```python
from build123d import *

# Parameters (mm, degrees)
SKETCH1_W           = 115
SKETCH1_H           = 150
SKETCH1_R           = 7.5
SKETCH1_W_2         = 15
SKETCH1_H_2         = 3
BOSS_EXTRUDE1_DEPTH = 3


with BuildPart() as part:
    # Sketch1 → Boss-Extrude1 (new body)
    with BuildSketch(Plane.XY):
        Rectangle(SKETCH1_W, SKETCH1_H)
        with Locations((0, -13.5)):
            Circle(SKETCH1_R, mode=Mode.SUBTRACT)
        with Locations((15, 70.5)):
            Rectangle(SKETCH1_W_2, SKETCH1_H_2, mode=Mode.SUBTRACT)
        with Locations((-40, 70.5)):
            Rectangle(SKETCH1_W_2, SKETCH1_H_2, mode=Mode.SUBTRACT)
        with Locations((-15, 70.5)):
            Rectangle(SKETCH1_W_2, SKETCH1_H_2, mode=Mode.SUBTRACT)
        with Locations((40, 70.5)):
            Rectangle(SKETCH1_W_2, SKETCH1_H_2, mode=Mode.SUBTRACT)
        with Locations((40, -70.5)):
            Rectangle(SKETCH1_W_2, SKETCH1_H_2, mode=Mode.SUBTRACT)
        with Locations((15, -70.5)):
            Rectangle(SKETCH1_W_2, SKETCH1_H_2, mode=Mode.SUBTRACT)
        with Locations((-15, -70.5)):
            Rectangle(SKETCH1_W_2, SKETCH1_H_2, mode=Mode.SUBTRACT)
        with Locations((-40, -70.5)):
            Rectangle(SKETCH1_W_2, SKETCH1_H_2, mode=Mode.SUBTRACT)
        with Locations((14.7, 43.5)):
            Rectangle(SKETCH1_W_2, SKETCH1_H_2, mode=Mode.SUBTRACT)
        with Locations((-39.7, 43.5)):
            Rectangle(SKETCH1_W_2, SKETCH1_H_2, mode=Mode.SUBTRACT)
        with Locations((-14.7, 43.5)):
            Rectangle(SKETCH1_W_2, SKETCH1_H_2, mode=Mode.SUBTRACT)
        with Locations((39.7, 43.5)):
            Rectangle(SKETCH1_W_2, SKETCH1_H_2, mode=Mode.SUBTRACT)
        with BuildLine():
            Line((39.5, -7.5), (39.5, 11.686291501))
            ThreePointArc((39.5, 11.686291501), (37.648050297, 14.457930099), (34.378679656, 13.807611845))
            Line((34.378679656, 13.807611845), (16.655175669, -3.915892143))
            ThreePointArc((16.655175669, -3.915892143), (16.374485428, -4.467252196), (16.471908992, -5.078229748))
            ThreePointArc((16.471908992, -5.078229748), (17.443347183, -7.33723771), (18.106599572, -9.705128205))
            ThreePointArc((18.106599572, -9.705128205), (18.454909512, -10.276250026), (19.085334684, -10.5))
            Line((19.085334684, -10.5), (36.5, -10.5))
            ThreePointArc((36.5, -10.5), (38.621320344, -9.621320344), (39.5, -7.5))
        make_face(mode=Mode.SUBTRACT)
        with BuildLine():
            Line((3, -32.585334684), (3, -50))
            ThreePointArc((3, -50), (3.878679656, -52.121320344), (6, -53))
            Line((6, -53), (25.186291501, -53))
            ThreePointArc((25.186291501, -53), (27.957930099, -51.148050297), (27.307611845, -47.878679656))
            Line((27.307611845, -47.878679656), (9.584107857, -30.155175669))
            ThreePointArc((9.584107857, -30.155175669), (9.032747804, -29.874485428), (8.421770252, -29.971908992))
            ThreePointArc((8.421770252, -29.971908992), (6.16276229, -30.943347183), (3.794871795, -31.606599572))
            ThreePointArc((3.794871795, -31.606599572), (3.223749974, -31.954909512), (3, -32.585334684))
        make_face(mode=Mode.SUBTRACT)
        with BuildLine():
            Line((16.655175669, -23.084107857), (34.378679656, -40.807611845))
            ThreePointArc((34.378679656, -40.807611845), (37.648050297, -41.457930099), (39.5, -38.686291501))
            Line((39.5, -38.686291501), (39.5, -19.5))
            ThreePointArc((39.5, -19.5), (38.621320344, -17.378679656), (36.5, -16.5))
            Line((36.5, -16.5), (19.085334684, -16.5))
            ThreePointArc((19.085334684, -16.5), (18.454909512, -16.723749974), (18.106599572, -17.294871795))
            ThreePointArc((18.106599572, -17.294871795), (17.443347183, -19.66276229), (16.471908992, -21.921770252))
            ThreePointArc((16.471908992, -21.921770252), (16.374485428, -22.532747804), (16.655175669, -23.084107857))
        make_face(mode=Mode.SUBTRACT)
        with BuildLine():
            Line((6, 26), (25.186291501, 26))
            ThreePointArc((25.186291501, 26), (27.957930099, 24.148050297), (27.307611845, 20.878679656))
            Line((27.307611845, 20.878679656), (9.584107857, 3.155175669))
            ThreePointArc((9.584107857, 3.155175669), (9.032747804, 2.874485428), (8.421770252, 2.971908992))
            ThreePointArc((8.421770252, 2.971908992), (6.16276229, 3.943347183), (3.794871795, 4.606599572))
            ThreePointArc((3.794871795, 4.606599572), (3.223749974, 4.954909512), (3, 5.585334684))
            Line((3, 5.585334684), (3, 23))
            ThreePointArc((3, 23), (3.878679656, 25.121320344), (6, 26))
        make_face(mode=Mode.SUBTRACT)
        with BuildLine():
            Line((-3, 5.585334684), (-3, 23))
            ThreePointArc((-3, 23), (-3.878679656, 25.121320344), (-6, 26))
            Line((-6, 26), (-25.186291501, 26))
            ThreePointArc((-25.186291501, 26), (-27.957930099, 24.148050297), (-27.307611845, 20.878679656))
            Line((-27.307611845, 20.878679656), (-9.584107857, 3.155175669))
            ThreePointArc((-9.584107857, 3.155175669), (-9.032747804, 2.874485428), (-8.421770252, 2.971908992))
            ThreePointArc((-8.421770252, 2.971908992), (-6.16276229, 3.943347183), (-3.794871795, 4.606599572))
            ThreePointArc((-3.794871795, 4.606599572), (-3.223749974, 4.954909512), (-3, 5.585334684))
        make_face(mode=Mode.SUBTRACT)
        with BuildLine():
            Line((-39.5, -7.5), (-39.5, 11.686291501))
            ThreePointArc((-39.5, 11.686291501), (-37.648050297, 14.457930099), (-34.378679656, 13.807611845))
            Line((-34.378679656, 13.807611845), (-16.655175669, -3.915892143))
            ThreePointArc((-16.655175669, -3.915892143), (-16.374485428, -4.467252196), (-16.471908992, -5.078229748))
            ThreePointArc((-16.471908992, -5.078229748), (-17.443347183, -7.33723771), (-18.106599572, -9.705128205))
            ThreePointArc((-18.106599572, -9.705128205), (-18.454909512, -10.276250026), (-19.085334684, -10.5))
            Line((-19.085334684, -10.5), (-36.5, -10.5))
            ThreePointArc((-36.5, -10.5), (-38.621320344, -9.621320344), (-39.5, -7.5))
        make_face(mode=Mode.SUBTRACT)
        with BuildLine():
            Line((-19.085334684, -16.5), (-36.5, -16.5))
            ThreePointArc((-36.5, -16.5), (-38.621320344, -17.378679656), (-39.5, -19.5))
            Line((-39.5, -19.5), (-39.5, -38.686291501))
            ThreePointArc((-39.5, -38.686291501), (-37.648050297, -41.457930099), (-34.378679656, -40.807611845))
            Line((-34.378679656, -40.807611845), (-16.655175669, -23.084107857))
            ThreePointArc((-16.655175669, -23.084107857), (-16.374485428, -22.532747804), (-16.471908992, -21.921770252))
            ThreePointArc((-16.471908992, -21.921770252), (-17.443347183, -19.66276229), (-18.106599572, -17.294871795))
            ThreePointArc((-18.106599572, -17.294871795), (-18.454909512, -16.723749974), (-19.085334684, -16.5))
        make_face(mode=Mode.SUBTRACT)
        with BuildLine():
            Line((-3, -32.585334684), (-3, -50))
            ThreePointArc((-3, -50), (-3.878679656, -52.121320344), (-6, -53))
            Line((-6, -53), (-25.186291501, -53))
            ThreePointArc((-25.186291501, -53), (-27.957930099, -51.148050297), (-27.307611845, -47.878679656))
            Line((-27.307611845, -47.878679656), (-9.584107857, -30.155175669))
            ThreePointArc((-9.584107857, -30.155175669), (-9.032747804, -29.874485428), (-8.421770252, -29.971908992))
            ThreePointArc((-8.421770252, -29.971908992), (-6.16276229, -30.943347183), (-3.794871795, -31.606599572))
            ThreePointArc((-3.794871795, -31.606599572), (-3.223749974, -31.954909512), (-3, -32.585334684))
        make_face(mode=Mode.SUBTRACT)
        with BuildLine():
            Line((12.657211383, 2.127059864), (38.658474042, 28.128322523))
            ThreePointArc((38.658474042, 28.128322523), (41.628322523, 28.128322523), (41.628322523, 25.158474042))
            Line((41.628322523, 25.158474042), (15.627059864, -0.842788617))
            ThreePointArc((15.627059864, -0.842788617), (12.657211383, -0.842788617), (12.657211383, 2.127059864))
        make_face(mode=Mode.SUBTRACT)
        with BuildLine():
            Line((12.657211383, -29.127059864), (38.658474042, -55.128322523))
            ThreePointArc((38.658474042, -55.128322523), (41.628322523, -55.128322523), (41.628322523, -52.158474042))
            Line((41.628322523, -52.158474042), (15.627059864, -26.157211383))
            ThreePointArc((15.627059864, -26.157211383), (12.657211383, -26.157211383), (12.657211383, -29.127059864))
        make_face(mode=Mode.SUBTRACT)
        with BuildLine():
            Line((-12.657211383, -29.127059864), (-38.658474042, -55.128322523))
            ThreePointArc((-38.658474042, -55.128322523), (-41.628322523, -55.128322523), (-41.628322523, -52.158474042))
            Line((-41.628322523, -52.158474042), (-15.627059864, -26.157211383))
            ThreePointArc((-15.627059864, -26.157211383), (-12.657211383, -26.157211383), (-12.657211383, -29.127059864))
        make_face(mode=Mode.SUBTRACT)
        with BuildLine():
            Line((-12.657211383, 2.127059864), (-38.658474042, 28.128322523))
            ThreePointArc((-38.658474042, 28.128322523), (-41.628322523, 28.128322523), (-41.628322523, 25.158474042))
            Line((-41.628322523, 25.158474042), (-15.627059864, -0.842788617))
            ThreePointArc((-15.627059864, -0.842788617), (-12.657211383, -0.842788617), (-12.657211383, 2.127059864))
        make_face(mode=Mode.SUBTRACT)
    extrude(amount=BOSS_EXTRUDE1_DEPTH)


solid = part.part
```
Design review of the part built by this model. Coordinates are the model's own, in mm. Coordinates: 2 decimals unless noted, no trailing zeros. Loops run counter-clockwise (first coordinate to the right, second up) from the corner with the lowest first, then second, coordinate; pieces in that order, holes last. Notation, with made-up numbers: (86.5, 13.5) - (145.5, 13.5) arc R29 ccw to (145.5, 42.5) - close; hole circle Ø11 at (33.25, -23.75). An arc over 180 degrees is marked (long way). Use CSV: the item, a comma, the result in double quotes. Start each with the question number.
1) Consider section C-C on y = 19. Write out the cut boundary in (x, z).
2) Consider section D-D on z = 0.5. Give the number of separate pieces and of enclosed holes in the cut face, then the cut area to 3 significant figures.
3) Wall thickness on L1, parallel to Y at x = -46, z = 1.55; L2, parallel to Y at x = -9, z = 0.2; L3, parallel to X at y = 21, z = 2.65: over which ranges is each line inside the solid? List them lowest first. Write a range as from..to.
4) Consider section A-A on y = -13.5. Write out the cut boundary in (x, z).
5) The part is to be moulded in two halves that separate along Y. For faces 1 (the flat face through (-1, 1, 3)), 2 (the cylindrical face through (38.64, -17.4, 1.48)), say which applies: +Y half, -Y half, draft (parallel to the pull), parting line (faces both ways), or undercut.
6) Consider section B-B on x = 0. Write out the cut boundary in (y, z).
7) For pin 1 Ø1.5 at (x, y) = (19.5, -18.5) entering from +Z; pin 2 Ø2 at (x, y) = (-43, 51.5) entering from -Z, all flat-tipped, find the tip position at first contact; note any pin that passes through.
Geometry says:
1,outline,"(-57.5, 0) - (-35.47, 0) - (-35.47, 3) - (-57.5, 3) - close; (-29.53, 0) - (-25.43, 0) - (-25.43, 3) - (-29.53, 3) - close; (-3, 0) - (3, 0) - (3, 3) - (-3, 3) - close; (25.43, 0) - (29.53, 0) - (29.53, 3) - (25.43, 3) - close; (35.47, 0) - (57.5, 0) - (57.5, 3) - (35.47, 3) - close"
2,separate pieces,"1"
2,enclosed holes,"25"
2,area,"12,700 mm^2"
3,L1,"-75..-72, -69..42, 45..69, 72..75"
3,L2,"-75..-72, -69..-53, -29.87..2.87, 26..42, 45..69, 72..75"
3,L3,"-57.5..-37.47, -31.53..-27.42, -3..3, 27.42..31.53, 37.47..57.5"
4,outline,"(-57.5, 0) - (-7.5, 0) - (-7.5, 3) - (-57.5, 3) - close; (7.5, 0) - (57.5, 0) - (57.5, 3) - (7.5, 3) - close"
5,face 1,"draft"
5,face 2,"undercut"
6,outline,"(-75, 0) - (-21, 0) - (-21, 3) - (-75, 3) - close; (-6, 0) - (75, 0) - (75, 3) - (-6, 3) - close"
7,pin 1,"through"
7,pin 2,"z = 0"
